```python
from build123d import *

# Parameters (mm, degrees)
SKETCH1_W               = 135
SKETCH1_H               = 90
SKETCH1_R               = 17.5
BOSS_EXTRUDE1_DEPTH     = 11
SKETCH3_R               = 9.5
CUT_EXTRUDE1_DEPTH      = 5
CUT_EXTRUDE2_DEPTH      = 82.867270628
CUT_EXTRUDE2_DEPTH_BACK = 82.867270628
SKETCH5_R               = 5
SKETCH6_R               = 8
CUT_EXTRUDE3_DEPTH      = 10
SKETCH7_W               = 135
SKETCH7_H               = 90
SKETCH7_W_2             = 110
SKETCH7_H_2             = 82
BOSS_EXTRUDE2_DEPTH     = 31
SKETCH8_W               = 135
SKETCH8_H               = 42
BOSS_EXTRUDE3_DEPTH     = 50
SKETCH9_W               = 120
SKETCH9_H               = 30
CUT_EXTRUDE4_DEPTH      = 35
SKETCH10_R              = 5
CUT_EXTRUDE5_DEPTH      = 101
SKETCH11_R              = 8
CUT_EXTRUDE6_DEPTH      = 10


with BuildPart() as part:
    # Sketch1 → Boss-Extrude1 (new body)
    with BuildSketch(Plane(origin=(0, 0, 0), x_dir=(1, 0, 0), z_dir=(0, 1, 0))):
        Rectangle(SKETCH1_W, SKETCH1_H)
        with Locations(Location((0, -22.5, 0), (0, 0, 270))):
            Circle(SKETCH1_R, mode=Mode.SUBTRACT)
    extrude(amount=BOSS_EXTRUDE1_DEPTH)

    # Sketch3 → Cut-Extrude1 (cut)
    with BuildSketch(Plane(origin=(0, 11, 0), x_dir=(1, 0, 0), z_dir=(0, 1, 0))):
        with Locations(Location((45, -22.5, 0), (0, 0, 270))):
            Circle(SKETCH3_R)
        with Locations(Location((-45, -22.5, 0), (0, 0, 270))):
            Circle(SKETCH3_R)
    extrude(amount=-CUT_EXTRUDE1_DEPTH, mode=Mode.SUBTRACT)

    # Sketch5 → Cut-Extrude2 (cut, two sides: drawn at the far end of the back side and taken through both)
    with BuildSketch(Plane(origin=(0, 11, 0), x_dir=(1, 0, 0), z_dir=(0, 1, 0)).offset(-CUT_EXTRUDE2_DEPTH_BACK)):
        with Locations(Location((0, 22.5, 0), (0, 0, 270))):
            Circle(SKETCH5_R)
        with Locations(Location((45, 22.5, 0), (0, 0, 270))):
            Circle(SKETCH5_R)
        with Locations(Location((-45, 22.5, 0), (0, 0, 270))):
            Circle(SKETCH5_R)
    extrude(amount=CUT_EXTRUDE2_DEPTH + CUT_EXTRUDE2_DEPTH_BACK, mode=Mode.SUBTRACT)

    # Sketch6 → Cut-Extrude3 (cut)
    with BuildSketch(Plane.XZ):
        with Locations(Location((45, -22.5, 0), (0, 0, 270))):
            Circle(SKETCH6_R)
        with Locations(Location((0, -22.5, 0), (0, 0, 270))):
            Circle(SKETCH6_R)
        with Locations(Location((-45, -22.5, 0), (0, 0, 90))):
            Circle(SKETCH6_R)
    extrude(amount=-CUT_EXTRUDE3_DEPTH, mode=Mode.SUBTRACT)

    # Sketch7 → Boss-Extrude2 (add)
    with BuildSketch(Plane.XZ):
        Rectangle(SKETCH7_W, SKETCH7_H)
        Rectangle(SKETCH7_W_2, SKETCH7_H_2, mode=Mode.SUBTRACT)
    extrude(amount=BOSS_EXTRUDE2_DEPTH)

    # Sketch8 → Boss-Extrude3 (add)
    with BuildSketch(Plane.XY.offset(45)):
        with Locations((0, -10)):
            Rectangle(SKETCH8_W, SKETCH8_H)
    extrude(amount=BOSS_EXTRUDE3_DEPTH)

    # Sketch9 → Cut-Extrude4 (cut)
    with BuildSketch(Plane.XY.offset(95)):
        with Locations((0, -10)):
            Rectangle(SKETCH9_W, SKETCH9_H)
    extrude(amount=-CUT_EXTRUDE4_DEPTH, mode=Mode.SUBTRACT)

    # Sketch10 → Cut-Extrude5 (cut)
    with BuildSketch(Plane.XY.offset(60)):
        with Locations((-40, -10)):
            Circle(SKETCH10_R)
        with Locations(Location((40, -10, 0), (0, 0, 180))):
            Circle(SKETCH10_R)
        with Locations((0, -10)):
            Circle(SKETCH10_R)
    extrude(amount=-CUT_EXTRUDE5_DEPTH, mode=Mode.SUBTRACT)

    # Sketch11 → Cut-Extrude6 (cut)
    with BuildSketch(Plane(origin=(0, 0, 41), x_dir=(-1, 0, 0), z_dir=(0, 0, -1))):
        with Locations((0, -10)):
            Circle(SKETCH11_R)
        with Locations((-40, -10)):
            Circle(SKETCH11_R)
        with Locations((40, -10)):
            Circle(SKETCH11_R)
    extrude(amount=-CUT_EXTRUDE6_DEPTH, mode=Mode.SUBTRACT)


solid = part.part
```
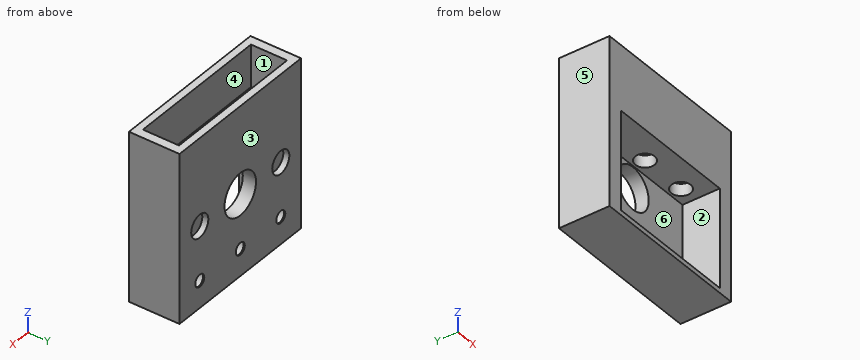
Here's how the part is built. I have some questions about the finished solid (model axes, mm). Face numbers are marked on the shaded views. A direction names the side the tool comes from. Give positions to 0.01 mm unless a question says otherwise; leave off trailing zeros. Write each loop counter-clockwise with the first axis right and the second up, starting at its lowest first coordinate (ties: lowest second). Pieces come first, ordered by that corner, then holes. Notation, with made-up numbers: (89.5, 62.5) -> (132.5, 62.5) arc R14 ccw to (132.5, 77.5) -> close; hole circle Ø5 at (40.5, 60). An arc over 180 degrees is marked (long way). Write each question's results on one line, items separated by ' | '.
Item 1: If I drill on L1, parallel to X at y = 5.25, z = -22.5; L2, parallel to Y at x = -40, z = 54.5; L3, parallel to X at y = -12, z = 28, over which ranges is the centre line in solid material (lowest first)?
Output:
L1: x = -67.5 to -53, -37 to -8, 8 to 37, 53 to 67.5 | L2: y = -31 to -15, -5 to 11 | L3: x = -67.5 to -55, 55 to 67.5
Item 2: On a 3-axis mill with a long thin cutter (end or side, diameter ignored), from which of +Z, -Z, +X, -X, +Y, -Y can I reach the whole of each face in a straight line? I mean the marked faces 4, 5 and 6. Say none if no direction works.
Output:
face 4: +Z | face 5: +Z, -Z, -X, +Y, -Y | face 6: -Y
Item 3: For pin 1 Ø3 at (x, z) = (4.5, -12.5) entering from -Y; pin 2 Ø8 at (x, y) = (0, -10) entering from +Z; pin 3 Ø13 at (x, z) = (49, -20.5) entering from -Y; pin 4 Ø5.5 at (x, z) = (41, 25) entering from +Y, each with a flat end and sliding along its axis, tell me the tip position at first contact or that it passes through.
Output:
pin 1: stops at y = 0 | pin 2: stops at z = -41 | pin 3: stops at y = -31 | pin 4: stops at y = 6
Item 4: Suppose I cut it at C-C on y = 2. Write out the boundary of the cut face in (x, z), plus the area to 3 significant figures.
Output:
outline: (-67.5, -45) -> (67.5, -45) -> (67.5, 95) -> (60, 95) -> (60, 60) -> (-60, 60) -> (-60, 95) -> (-67.5, 95) -> close; hole circle Ø16 at (-45, -22.5); hole circle Ø35 at (0, 22.5); hole circle Ø16 at (0, -22.5); hole circle Ø16 at (45, -22.5) | area: 13,100 mm^2
Item 5: Suppose I cut it at D-D on z = 22.5. Write out the boundary of the cut face in (x, y), plus the area to 4 significant figures.
Output:
outline: (-67.5, -31) -> (-55, -31) -> (-55, 0) -> (-17.5, 0) -> (-17.5, 11) -> (-35.5, 11) -> (-35.5, 6) -> (-54.5, 6) -> (-54.5, 11) -> (-67.5, 11) -> close; (17.5, 0) -> (55, 0) -> (55, -31) -> (67.5, -31) -> (67.5, 11) -> (54.5, 11) -> (54.5, 6) -> (35.5, 6) -> (35.5, 11) -> (17.5, 11) -> close | area: 1,685 mm^2
Item 6: Suppose I cut it at A-A on z = -22.5. Give the number of separate pieces and of enclosed holes in the cut face, plus the area to 3 significant figures.
Output:
separate pieces: 4 | enclosed holes: 0 | area: 1,750 mm^2
Item 7: We'd pull the mould along Y, two halves only. Please class the marked faces 1, 2 and 3: pulls with the +Y half, pulls with the -Y half, needs draft (parallel to the pull), parting line crosses it, or undercut.
Output:
face 1: undercut | face 2: needs draft | face 3: pulls with the +Y half
